from build123d import *

# Parameters (mm, degrees)
SKETCH1_W               = 8
SKETCH1_H               = 8
BOSS_EXTRUDE1_DEPTH     = 3
CUT_EXTRUDE1_DEPTH      = 12.704699911
CUT_EXTRUDE1_DEPTH_BACK = 12.704699911
CUT_EXTRUDE2_DEPTH      = 11
SKETCH4_R               = 1.8
CUT_EXTRUDE3_DEPTH      = 0.8
SKETCH5_W               = 8
SKETCH5_H               = 1
BOSS_EXTRUDE2_DEPTH     = 2
FILLET1_R               = 4
CUT_EXTRUDE4_DEPTH      = 0.4
CUT_EXTRUDE5_DEPTH      = 0.4


with BuildPart() as part:
    # Sketch1 → Boss-Extrude1 (new body)
    with BuildSketch(Plane(origin=(0, 0, 0), x_dir=(1, 0, 0), z_dir=(0, 1, 0))):
        with Locations((4, 4)):
            Rectangle(SKETCH1_W, SKETCH1_H)
    extrude(amount=BOSS_EXTRUDE1_DEPTH)

    # Sketch2 → Cut-Extrude1 (cut, two sides: drawn at the far end of the back side and taken through both)
    with BuildSketch(Plane.XY.offset(-CUT_EXTRUDE1_DEPTH_BACK)):
        Polygon((0, 0), (0.6, 3), (0, 3), align=None)
        Polygon((8, 0), (7.4, 3), (8, 3), align=None)
    extrude(amount=CUT_EXTRUDE1_DEPTH + CUT_EXTRUDE1_DEPTH_BACK, mode=Mode.SUBTRACT)

    # Sketch3 → Cut-Extrude2 (cut)
    with BuildSketch(Plane(origin=(0, 0, 0), x_dir=(0, 0, -1), z_dir=(1, 0, 0))):
        Polygon((0, 0), (0.6, 3), (0, 3), align=None)
        Polygon((8, 3), (7.4, 3), (8, 0), align=None)
    extrude(amount=CUT_EXTRUDE2_DEPTH, mode=Mode.SUBTRACT)

    # Sketch4 → Cut-Extrude3 (cut)
    with BuildSketch(Plane.XZ):
        with Locations(Location((4, -3.75, 0), (0, 0, 270))):
            Circle(SKETCH4_R)
    extrude(amount=-CUT_EXTRUDE3_DEPTH, mode=Mode.SUBTRACT)

    # Sketch5 → Boss-Extrude2 (add)
    with BuildSketch(Plane.XZ):
        with Locations((4, -7.5)):
            Rectangle(SKETCH5_W, SKETCH5_H)
    extrude(amount=BOSS_EXTRUDE2_DEPTH)

    # Fillet1
    # the kernel refuses this fillet: 4 mm, written as the material it takes off along each edge
    with BuildSketch(Plane(origin=(8, -2, -16.660254038), x_dir=(0, 1, 0), z_dir=(0, 0, 1)), Plane(origin=(0, -2, 1.660254038), x_dir=(0, 1, 0), z_dir=(0, 0, -1))) as fillet1_piece_1:
        with BuildLine():
            CenterArc((4, 3.464101615), FILLET1_R, 180, 60)
            Line((0, 3.464101615), (-0.08, 3.464101615))
            Line((-0.08, 3.464101615), (-0.08, 0))
            Line((-0.08, 0), (0, -0.08))
            ThreePointArc((0, -0.08), (1, -0.08), (1.96, -0.069282032))
            Line((1.96, -0.069282032), (2, 0))
        make_face()
    extrude(amount=18.320508076, mode=Mode.SUBTRACT)

    # Sketch6 → Cut-Extrude4 (cut)
    with BuildSketch(Plane(origin=(0, 3, 0), x_dir=(1, 0, 0), z_dir=(0, 1, 0))):
        Polygon((3.652362984, 2.002856352), (3.652362984, 5.336189685), (2.472875805, 5.336189685), (2.472875805, 6.002856352), (5.601080933, 6.002856352), (5.601080933, 5.336189685), (4.421593754, 5.336189685), (4.421593754, 2.002856352), align=None)
    extrude(amount=-CUT_EXTRUDE4_DEPTH, mode=Mode.SUBTRACT)

    # Sketch7 → Cut-Extrude5 (cut)
    with BuildSketch(Plane(origin=(0, 3, 0), x_dir=(1, 0, 0), z_dir=(0, 1, 0))):
        with BuildLine():
            Line((5.873519392, 1.453659702), (6.173519392, 1.492602009))
            add(Edge.make_bspline(
                [(6.173519392, 1.492602009), (6.1768382, 1.472256976), (6.18322911, 1.433079261), (6.203068429, 1.378384162), (6.230697403, 1.330199963), (6.266205672, 1.289626965), (6.30661854, 1.256629271), (6.351264588, 1.233104776), (6.398791495, 1.218293755), (6.431707248, 1.216554551), (6.448279008, 1.215678932)],
                knots=[0, 0, 0, 0, 1.154848647, 2.223851388, 3.245409892, 4.254330626, 5.232966172, 6.156270698, 7.071756339, 8, 8, 8, 8], degree=3))
            add(Edge.make_bspline(
                [(6.448279008, 1.215678932), (6.457906388, 1.215848075), (6.476752132, 1.216179174), (6.504524052, 1.219937575), (6.531053869, 1.226043662), (6.55659259, 1.234330756), (6.580874213, 1.245230043), (6.603920328, 1.258567919), (6.625817059, 1.274363121), (6.646675237, 1.292223374), (6.665948362, 1.312615024), (6.682055884, 1.336087325), (6.696325112, 1.361440746), (6.707949377, 1.389364059), (6.716328852, 1.41995512), (6.722995329, 1.45269023), (6.726393576, 1.487964606), (6.7270346, 1.51218758), (6.727365546, 1.524693355)],
                knots=[0, 0, 0, 0, 0.981268084, 1.920847364, 2.851509818, 3.754644372, 4.654445699, 5.560569672, 6.465366234, 7.403985617, 8.358004942, 9.316972086, 10.299158387, 11.321223707, 12.392031981, 13.529051644, 14.724304971, 16, 16, 16, 16], degree=3))
            add(Edge.make_bspline(
                [(6.727365546, 1.524693355), (6.727178419, 1.536481523), (6.726816764, 1.559264099), (6.723461454, 1.592272205), (6.718311073, 1.623118586), (6.710117629, 1.651577708), (6.700760071, 1.678178631), (6.688143723, 1.701978526), (6.674300374, 1.724011312), (6.657427434, 1.743088207), (6.639042824, 1.759943867), (6.619463278, 1.774961982), (6.598469004, 1.787493154), (6.576269045, 1.79824857), (6.552478567, 1.806082762), (6.527290541, 1.811294815), (6.501043648, 1.815207497), (6.483029864, 1.815520133), (6.473879969, 1.815678932)],
                knots=[0, 0, 0, 0, 1.29221626, 2.497420946, 3.635005972, 4.715822244, 5.741640361, 6.720139245, 7.663294346, 8.588224307, 9.502291809, 10.395891443, 11.288713187, 12.178904539, 13.095818132, 14.026458458, 14.997562253, 16, 16, 16, 16], degree=3))
            add(Edge.make_bspline(
                [(6.473879969, 1.815678932), (6.462311673, 1.815264192), (6.439232742, 1.814436778), (6.405164091, 1.807710713), (6.372003678, 1.796760631), (6.339785969, 1.781517356), (6.308596201, 1.761859078), (6.278569411, 1.737720606), (6.249190173, 1.70951724), (6.23114374, 1.688207441), (6.2218367, 1.677217394)],
                knots=[0, 0, 0, 0, 0.931687088, 1.85873035, 2.786835662, 3.740075265, 4.723687035, 5.750832598, 6.840042753, 8, 8, 8, 8], degree=3))
            Line((6.2218367, 1.677217394), (5.919673238, 1.719765471))
            Line((5.919673238, 1.719765471), (6.127365546, 2.715678932))
            Line((6.127365546, 2.715678932), (7.004288623, 2.715678932))
            Line((7.004288623, 2.715678932), (7.004288623, 2.369525086))
            Line((7.004288623, 2.369525086), (6.405009777, 2.369525086))
            Line((6.405009777, 2.369525086), (6.3343367, 2.048251048))
            add(Edge.make_bspline(
                [(6.3343367, 2.048251048), (6.352346227, 2.058641979), (6.3874181, 2.078877348), (6.443410579, 2.099707804), (6.499690691, 2.113077126), (6.537629531, 2.114816152), (6.556452085, 2.115678932)],
                knots=[0, 0, 0, 0, 1.060051984, 2.064352337, 3.039669322, 4, 4, 4, 4], degree=3))
            add(Edge.make_bspline(
                [(6.556452085, 2.115678932), (6.574146885, 2.115202759), (6.60910097, 2.114262131), (6.660364054, 2.106544582), (6.709535097, 2.093825268), (6.756780138, 2.076125011), (6.801761249, 2.052924592), (6.844866196, 2.024883357), (6.885472675, 1.991514713), (6.924016987, 1.953782044), (6.959166694, 1.912035385), (6.989521263, 1.866512768), (7.015738821, 1.818347997), (7.037083021, 1.767008911), (7.053155816, 1.712424088), (7.065192785, 1.655063547), (7.07193581, 1.594565079), (7.072984339, 1.553314949), (7.073519392, 1.532265471)],
                knots=[0, 0, 0, 0, 0.974409932, 1.924837087, 2.848242317, 3.768103797, 4.697919751, 5.630842317, 6.595644344, 7.588240789, 8.59876155, 9.595918743, 10.597287627, 11.615415169, 12.652315553, 13.727511434, 14.840374562, 16, 16, 16, 16], degree=3))
            add(Edge.make_bspline(
                [(7.073519392, 1.532265471), (7.073036469, 1.514585649), (7.072077961, 1.479494734), (7.066471429, 1.42756738), (7.056005109, 1.377169317), (7.042672536, 1.328016631), (7.024246745, 1.280521142), (7.002381003, 1.234373213), (6.976242653, 1.189655711), (6.956076521, 1.161441782), (6.945875162, 1.147169317)],
                knots=[0, 0, 0, 0, 1.027524957, 2.039431707, 3.02972907, 4.015954419, 4.995255842, 5.985553205, 6.980960039, 8, 8, 8, 8], degree=3))
            add(Edge.make_bspline(
                [(6.945875162, 1.147169317), (6.931003624, 1.128791302), (6.901734709, 1.092621232), (6.851630217, 1.045066578), (6.797135444, 1.00512898), (6.738397987, 0.97233011), (6.675480422, 0.946591981), (6.608098871, 0.928697649), (6.536747385, 0.917626673), (6.487743367, 0.916337636), (6.462702085, 0.915678932)],
                knots=[0, 0, 0, 0, 1.018121711, 2.003781959, 2.967346956, 3.92281574, 4.896313303, 5.889026666, 6.921282725, 8, 8, 8, 8], degree=3))
            add(Edge.make_bspline(
                [(6.462702085, 0.915678932), (6.442489279, 0.916044029), (6.403022672, 0.9167569), (6.345224712, 0.92380666), (6.290451314, 0.935259909), (6.238356922, 0.95115359), (6.18925085, 0.971795666), (6.142751555, 0.99671717), (6.099246456, 1.026470486), (6.058935891, 1.060830838), (6.021919655, 1.09880899), (5.988902802, 1.140363971), (5.959526451, 1.184800784), (5.934351052, 1.232568443), (5.912895663, 1.28333195), (5.895811978, 1.337351468), (5.881746134, 1.394266746), (5.876291993, 1.433642912), (5.873519392, 1.453659702)],
                knots=[0, 0, 0, 0, 1.098912142, 2.145685936, 3.161086862, 4.139124218, 5.10307886, 6.053641493, 7.003731987, 7.963777669, 8.929946266, 9.883471279, 10.846206077, 11.822909928, 12.81603559, 13.839338588, 14.901632394, 16, 16, 16, 16], degree=3))
        make_face()
    extrude(amount=-CUT_EXTRUDE5_DEPTH, mode=Mode.SUBTRACT)


solid = part.part
The listing builds one solid part. Answer for the finished solid, in the listing's coordinates (mm). A direction names the side the tool comes from. Round coordinates to 2 decimals unless told otherwise and drop trailing zeros. Write each loop counter-clockwise with the first axis right and the second up, starting at its lowest first coordinate (ties: lowest second). Pieces come first, ordered by that corner, then holes. Notation, with made-up numbers: (3.5, 24.25) - (53.5, 24.25) arc R24 ccw to (53.5, 48.25) - close; hole circle Ø4 at (-13.5, 32.25). An arc over 180 degrees is marked (long way). Use one line per item in the form item = value. Start each with the question number.
Item 1: A cutting plane is placed at B-B (x = 4). Write down the section's boundary in (y, z).
Item 2: A cutting plane is placed at D-D (z = -3.75). Write down the section's boundary in (x, y), plus the area to 3 significant figures.
Item 3: A cutting plane is placed at A-A (z = -5.75). Write down the section's boundary in (x, y), plus the area to 3 significant figures.
Item 4: A cutting plane is placed at C-C (y = 2.3). Write down the section's boundary in (x, z).
Item 5: Find the intervals of material crossed by line 1 (Y direction, x = 5.25, z = -4.5); line 2 (Z direction, x = 4.25, y = -0.1); line 3 (Y direction, x = 4.5, z = -0.75), in increasing order. Write a range as [from, to].
Item 6: Flat-ended cylindrical pins translate along their axes: pin 1 Ø4 at (x, z) = (3, -4.5) entering from -Y; pin 2 Ø2 at (y, z) = (2.5, -5) entering from -X; pin 3 Ø0.6 at (x, y) = (2.5, -0.5) entering from +Z. Find the tip coordinate at first contact, or state that the pin passes through.
Item 7: A tool of negligible diameter and unlimited length cuts with its end or side. For faces 5 (the flat face through (3, 0, -2)), 6 (the flat face through (4, -1, -8)), from which of +Z, -Z, +X, -X, +Y, -Y can it reach the whole face along a straight path? Write none if from no direction.
Item 8: Determine the mould class of faces 1 (the cylindrical face through (4.541, 0.394, -5.467)), 2 (the cylindrical face through (6.51, -1.48, -7.51)), 3 (the flat face through (3.9, 1.5, -7.7)), 4 (the flat face through (4, 0.8, -4)) for opening direction X: +X half, -X half, draft (parallel to the pull), parting line (faces both ways), or undercut.
The answers:
q1.outline = (-2, -8) - (0, -8) - (3, -7.4) - (3, -6) - (2.6, -6) - (2.6, -2) - (3, -2) - (3, -0.6) - (0, 0) - (0, -1.95) - (0.8, -1.95) - (0.8, -5.55) - (0, -5.55) - (0, -7) - (-2, -7) - close
q2.outline = (0, 0) - (2.2, 0) - (2.2, 0.8) - (5.8, 0.8) - (5.8, 0) - (8, 0) - (7.4, 3) - (4.42, 3) - (4.42, 2.6) - (3.65, 2.6) - (3.65, 3) - (0.6, 3) - close
q2.area = 19.0 mm^2
q3.outline = (0, 0) - (8, 0) - (7.4, 3) - (5.6, 3) - (5.6, 2.6) - (2.47, 2.6) - (2.47, 3) - (0.6, 3) - close
q3.area = 20.9 mm^2
q4.outline = (0.46, -7.54) - (7.54, -7.54) - (7.54, -0.46) - (0.46, -0.46) - close
q5.line_1 = [0.8, 3]
q5.line_2 = [-8, -7]
q5.line_3 = [0, 3]
q6.pin_1 = 0
q6.pin_2 = 0.3
q6.pin_3 = -7
q7.face_5 = +Z, +X, -X, -Y
q7.face_6 = -Z, +X, -X, +Y, -Y
q8.face_1 = undercut
q8.face_2 = +X half
q8.face_3 = draft
q8.face_4 = undercut
